Study the drawing (mm; zero at the part's minimum x, y, z) and answer. A direction names the side the tool comes from. Give positions to 0.01 mm unless a question says otherwise; leave off trailing zeros. Write each loop counter-clockwise with the first axis right and the second up, starting at its lowest first coordinate (ties: lowest second). Pieces come first, ordered by that corner, then holes. Notation, with made-up numbers: (50, -10) - (57, -10) arc R18 ccw to (57, 10) - close; hole circle Ø3 at (-19.75, -2.5). An arc over 180 degrees is marked (long way). Return JSON: item names as keys, results as strings.
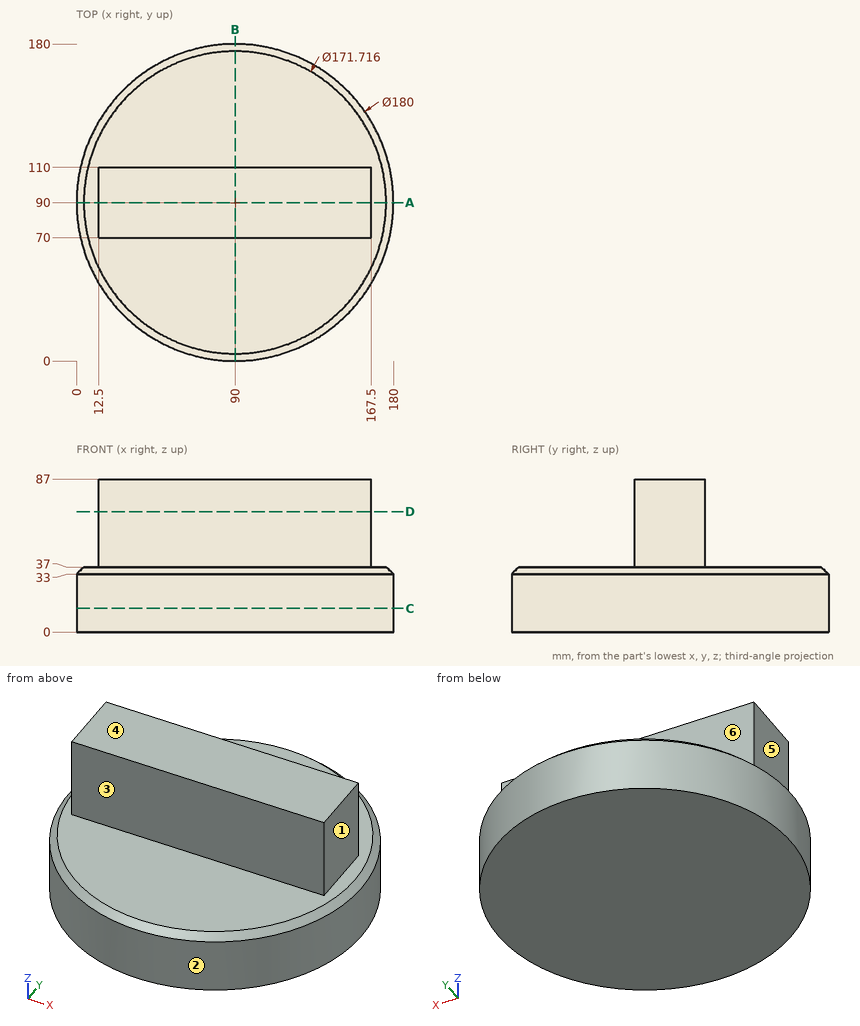
Item 1: Flat-ended cylindrical pins translate along their axes: P1, Ø4, axis at x = 57.5, z = 14.5, coming from the -Y side; P2, Ø3, axis at x = 53, z = 19, coming from the +Y side; P3, Ø8, axis at x = 154, z = 21.5, coming from the -Y side. Find the tip coordinate at first contact, or state that the pin passes through.
Answer below:
{"P1": "stops at y = 5.33", "P2": "stops at y = 172.7", "P3": "stops at y = 22.92"}
Item 2: The mould has two halves that part along X. Classify the marked faces 1, 2 and 3: +X half, -X half, draft (parallel to the pull), parting line (faces both ways), or undercut.
Answer below:
{"face 1": "+X half", "face 2": "parting line", "face 3": "draft"}
Item 3: A cutting plane is placed at D-D on z = 68.5. Determine the outline of the cut face in (x, y).
Answer below:
{"outline": "(12.5, 70) - (167.5, 70) - (167.5, 110) - (12.5, 110) - close"}
Item 4: For the marked faces 4, 5 and 6, determine the directions among +Z, -Z, +X, -X, +Y, -Y from which every point of the face is accessible in a straight line to the end or side of a thin tool.
Answer below:
{"face 4": "+Z, +X, -X, +Y, -Y", "face 5": "+Z, -X, +Y, -Y", "face 6": "+Z, +X, -X, +Y"}
Item 5: A cutting plane is placed at A-A on y = 90. Determine the outline of the cut face in (x, z).
Answer below:
{"outline": "(0, 0) - (180, 0) - (180, 33) - (175.86, 37) - (167.5, 37) - (167.5, 87) - (12.5, 87) - (12.5, 37) - (4.14, 37) - (0, 33) - close"}
Item 6: A cutting plane is placed at B-B on x = 90. Determine the outline of the cut face in (y, z), then the cut area to 3 significant figures.
Answer below:
{"outline": "(0, 0) - (180, 0) - (180, 33) - (175.86, 37) - (110, 37) - (110, 87) - (70, 87) - (70, 37) - (4.14, 37) - (0, 33) - close", "area": "8,640 mm²"}
Item 7: A cutting plane is placed at C-C on z = 13.5. Determine the outline of the cut face in (x, y).
Answer below:
{"outline": "circle Ø180 at (90, 90)"}
Item 8: Consider L1, parallel to Z at x = 63, y = 131; L2, parallel to Y at x = 140, z = 65; L3, parallel to X at y = 107.5, z = 69. Determine where each line is inside the solid, lowest interval first.
Answer below:
{"L1": "z = 0 to 37", "L2": "y = 70 to 110", "L3": "x = 12.5 to 167.5"}
